Build history of the part. All positions in model axes, mm. A direction names the side the tool comes from. Give positions to 0.01 mm unless a question says otherwise; leave off trailing zeros. Write each loop counter-clockwise with the first axis right and the second up, starting at its lowest first coordinate (ties: lowest second). Pieces come first, ordered by that corner, then holes. Notation, with made-up numbers: M -3.5,-39 L 40.5,-39 A35 ccw 40.5,0 Z; hole C 54.25,-36 d7. An arc over 180 degrees is marked long. One line per item, written item: value. Start each with the question number.
from build123d import *

# Parameters (mm, degrees)
F0_W     = 9
F0_H     = 9
F0_W_2   = 7
F0_H_2   = 7
F1_DEPTH = 10
F2_R     = 1.25
F3_DEPTH = 1
F4_R     = 2.5
F4_R_2   = 2.05
F5_DEPTH = 4
F7_DEPTH = 9


with BuildPart() as f1:
    # F0 (on Front) → F1 (new body)
    with BuildSketch(Plane.XZ):
        Rectangle(F0_W, F0_H)
        Rectangle(F0_W_2, F0_H_2, mode=Mode.SUBTRACT)
    extrude(amount=F1_DEPTH)

    # F2 (on face) → F3 (cut, through all)
    with BuildSketch(Plane.XY.offset(4.5)):
        with Locations((0, -5)):
            Circle(F2_R)
    extrude(amount=-F3_DEPTH, mode=Mode.SUBTRACT)

    # F4 (on face) → F5 (join)
    with BuildSketch(Plane.XY.offset(4.5)):
        with Locations((0, -5)):
            Circle(F4_R)
        with Locations((0, -5)):
            Circle(F4_R_2, mode=Mode.SUBTRACT)
    extrude(amount=F5_DEPTH)

    # F6 (on face) → F7 (join, through all)
    with BuildSketch(Plane.XY.offset(4.5)):
        with BuildLine():
            Line((-4.5, -2), (-4.5, 0))
            Line((-4.5, 0), (-5.5, 0))
            ThreePointArc((-5.5, 0), (-5.7928932188, -0.7071067812), (-6.5, -1))
            Line((-6.5, -1), (-6.5, -2))
            Line((-6.5, -2), (-4.5, -2))
        make_face()
        with BuildLine():
            Line((5.5, 0), (4.5, 0))
            Line((4.5, 0), (4.5, -2))
            Line((4.5, -2), (6.5, -2))
            Line((6.5, -2), (6.5, -1))
            ThreePointArc((6.5, -1), (5.7928932188, -0.7071067812), (5.5, 0))
        make_face()
    extrude(amount=-F7_DEPTH)

    # F8: F1 across face


with BuildPart() as f1_1:
    add(f1.part)
    add(f1.part.mirror(Plane(origin=(0, 0, 0), x_dir=(-1, 0, 0), z_dir=(0, 1, 0))))


solid = f1_1.part
1) Band-saw the part on D-D (y = -5). List the corners of the cut face in (x, z).
2) Band-saw the part on A-A (z = 2.5). List the corners of the cut face in (x, y), then the cut area to 3 significant figures.
3) Band-saw the part on B-B (x = 0). Count the separate pieces of the cut face and the enclosed holes in it, then the cut area to 3 significant figures.
4) Mould opens along X. For faces 1 (the face through (-2, 4, 8.5)), 2 (the face through (4.5, -6, 0)), 3 (the face through (-1, 6, 4.5)) say: released by +X, released by -X, zero draft, split by the parting line, or undercut.
5) Probe line 1 along Y through (x, z) = (0, 4); line 2 along Y through (x, z) = (-0.75, 5.75); line 3 along X through (y, z) = (8.25, -2). List the from-to ranges inside material, lowest first. Write a range as from..to.
6) Tool access for faces 4 (the face through (-6.5, -1.5, 0.1)), 5 (the face through (-0.33, 2.52, 6.47)), 6 (the face through (-6, 2, 0)), 7 (the face through (0, 0, -3.5)): list every direction of +Z, -Z, +X, -X, +Y, -Y with a clear straight run to the whole face (end or side of a thin tool).
7) Band-saw the part on C-C (y = 1.5). List the corners of the cut face in (x, z), then the cut area to 3 significant figures.
8) Drop flat-ended pins along their axis: P1, Ø2.5, axis at y = -7, z = -1, coming from the -X side; P2, Ø4, axis at y = 7.5, z = 0.5, coming from the +X side; P3, Ø2, axis at y = 8, z = 7, coming from the -X side; P4, Ø1.5, axis at x = 0.5, z = 2, coming from the -Y side. Give the stop position or say it passes through.
Model answer:
1. outline: M -4.5,-4.5 L 4.5,-4.5 L 4.5,4.5 L 2.5,4.5 L 2.5,8.5 L 2.05,8.5 L 2.05,4.5 L 1.25,4.5 L 1.25,3.5 L 3.5,3.5 L 3.5,-3.5 L -3.5,-3.5 L -3.5,3.5 L -1.25,3.5 L -1.25,4.5 L -2.05,4.5 L -2.05,8.5 L -2.5,8.5 L -2.5,4.5 L -4.5,4.5 Z
2. outline: M -6.5,-2 L -4.5,-2 L -4.5,-10 L -3.5,-10 L -3.5,10 L -4.5,10 L -4.5,2 L -6.5,2 L -6.5,1 A1 cw -6.5,-1 Z; M 3.5,-10 L 4.5,-10 L 4.5,-2 L 6.5,-2 L 6.5,-1 A1 cw 6.5,1 L 6.5,2 L 4.5,2 L 4.5,10 L 3.5,10 Z
2. area: 52.9 mm²
3. separate pieces: 4
3. enclosed holes: 0
3. area: 42.2 mm²
4. face 1: zero draft
4. face 2: released by +X
4. face 3: undercut
5. line 1: y = -10..-6.25, -3.75..3.75, 6.25..10
5. line 2: y = -7.38..-6.91, -3.09..-2.62, 2.62..3.09, 6.91..7.38
5. line 3: x = -4.5..-3.5, 3.5..4.5
6. face 4: +Z, -Z, -X, +Y, -Y
6. face 5: +Z
6. face 6: +Z, -Z, -X, +Y
6. face 7: +Y, -Y
7. outline: M -6.5,-4.5 L 6.5,-4.5 L 6.5,4.5 L -6.5,4.5 Z; hole M -3.5,-3.5 L 3.5,-3.5 L 3.5,3.5 L -3.5,3.5 Z
7. area: 68.0 mm²
8. P1: stops at x = -4.5
8. P2: stops at x = 4.5
8. P3: stops at x = -1.5
8. P4: passes through
